Check sheet for the modelled part. Datum: model origin and axes. Units: mm. Face numbers are marked on the shaded views. A direction names the side the tool comes from. Round coordinates to 2 decimals unless told otherwise and drop trailing zeros. Order: outer loops, then holes, each group sorted by start corner. A loop starts at its lowest first (then second) coordinate and runs counter-clockwise, first axis right, second up.
(1) Sectioned sample at B-B, the plane x = 9. Enter the section's corners in (y, z), and give its area (3 significant figures).
(2) Sectioned sample at C-C, the plane y = 61.5. Enter the section's corners in (x, z).
(3) Depth check by flat-ended pin: pin 1 (6 mm diameter, centred on x = 47, z = -31, fed in from +Y); pin 2 (8.5 mm diameter, centred on x = 9, y = 15.5, fed in from -Z); pin 3 (3 mm diameter, centred on x = 46.5, y = 28.5, fed in from -Z). Enter the tip coordinate at first touch or a pass-through.
(4) Sectioned sample at D-D, the plane x = 32.5. Enter the section's corners in (y, z), and give its area (3 significant figures).
(5) Tool access check on the marked faces 1 and 2. Record the directions out of +Z, -Z, +X, -X, +Y, -Y that give a thin tool (end or side, any length) a straight path to the whole face; none if there is none.
(6) Sectioned sample at A-A, the plane z = -20. Enter the section's corners in (x, y), and give its area (3 significant figures).
(7) Thickness scan on probe 1 along Z at (x, y) = (39, 6); probe 2 along Y at (x, z) = (20, -50); probe 3 along Y at (x, z) = (9, -0.85). Record the ranges inside material, lowest first.
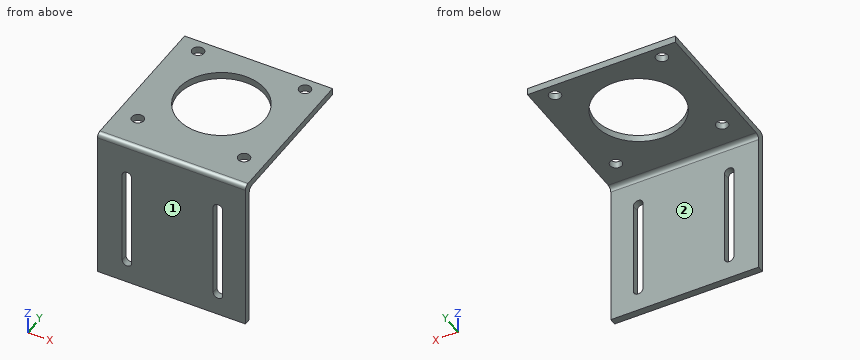
```python
from build123d import *

# Parameters (mm, degrees)
EXTRUDE_1_DEPTH     = 65
CUT_EXTRUDE_1_DEPTH = 115.341593482
SKETCH_3_R          = 19.1
SKETCH_3_R_2        = 2.6
CUT_EXTRUDE_2_DEPTH = 117.073252733


with BuildPart() as part:
    # Эскиз1 → Бобышка-Вытянуть1 (new body)
    with BuildSketch(Plane(origin=(0, 0, 0), x_dir=(0, 0, -1), z_dir=(1, 0, 0))):
        with BuildLine():
            Line((0, 68), (0, 2))
            ThreePointArc((0, 2), (0.585786438, 0.585786438), (2, 0))
            Line((2, 0), (68, 0))
            Line((68, 0), (68, 3))
            Line((68, 3), (5, 3))
            ThreePointArc((5, 3), (3.585786438, 3.585786438), (3, 5))
            Line((3, 5), (3, 68))
            Line((3, 68), (0, 68))
        make_face()
    extrude(amount=EXTRUDE_1_DEPTH)

    # Эскиз2 → Вырез-Вытянуть1 (cut, through all)
    with BuildSketch(Plane(origin=(0, 3, 0), x_dir=(1, 0, 0), z_dir=(0, 1, 0))):
        with BuildLine():
            Line((55.045453811, 58), (55.045453811, 16))
            ThreePointArc((55.045453811, 16), (52.945453811, 13.9), (50.845453811, 16))
            Line((50.845453811, 16), (50.845453811, 58))
            ThreePointArc((50.845453811, 58), (52.945453811, 60.1), (55.045453811, 58))
        make_face()
        with BuildLine():
            Line((10.845453811, 58), (10.845453811, 16))
            ThreePointArc((10.845453811, 16), (12.945453811, 13.9), (15.045453811, 16))
            Line((15.045453811, 16), (15.045453811, 58))
            ThreePointArc((15.045453811, 58), (12.945453811, 60.1), (10.845453811, 58))
        make_face()
    extrude(amount=-CUT_EXTRUDE_1_DEPTH, mode=Mode.SUBTRACT)

    # Эскиз3 → Вырез-Вытянуть2 (cut, through all)
    with BuildSketch(Plane.XY):
        with Locations((32.5, 39)):
            Circle(SKETCH_3_R)
        with Locations((9, 62.5)):
            Circle(SKETCH_3_R_2)
        with Locations((56, 62.5)):
            Circle(SKETCH_3_R_2)
        with Locations((55.996600846, 14.934748787)):
            Circle(SKETCH_3_R_2)
        with Locations((9, 15.5)):
            Circle(SKETCH_3_R_2)
    extrude(amount=-CUT_EXTRUDE_2_DEPTH, mode=Mode.SUBTRACT)


solid = part.part
```
Derived:
1. outline: (0, -68) - (3, -68) - (3, -5) arc R2 cw to (5, -3) - (12.9, -3) - (12.9, 0) - (2, 0) arc R2 ccw to (0, -2) - close; (18.1, -3) - (59.9, -3) - (59.9, 0) - (18.1, 0) - close; (65.1, -3) - (68, -3) - (68, 0) - (65.1, 0) - close
1. area: 368 mm2
2. outline: (0, -3) - (6.6, -3) - (6.6, 0) - (0, 0) - close; (11.4, -3) - (53.6, -3) - (53.6, 0) - (11.4, 0) - close; (58.4, -3) - (65, -3) - (65, 0) - (58.4, 0) - close
3. pin 1: stops at y = 3
3. pin 2: stops at z = -3
3. pin 3: passes through
4. outline: (0, -68) - (3, -68) - (3, -5) arc R2 cw to (5, -3) - (19.9, -3) - (19.9, 0) - (2, 0) arc R2 ccw to (0, -2) - close; (58.1, -3) - (68, -3) - (68, 0) - (58.1, 0) - close
4. area: 284 mm2
5. face 1: +Z, -Z, +X, -X, -Y
5. face 2: -Z, +X, -X, +Y
6. outline: (0, 0) - (10.85, 0) - (10.85, 3) - (0, 3) - close; (15.05, 0) - (50.85, 0) - (50.85, 3) - (15.05, 3) - close; (55.05, 0) - (65, 0) - (65, 3) - (55.05, 3) - close
6. area: 170 mm2
7. probe 1: z = -3 to 0
7. probe 2: y = 0 to 3
7. probe 3: y = 0.36 to 12.9, 18.1 to 59.9, 65.1 to 68
